Input: part model. Units: mm. Frame: model coordinates. A direction names the side the tool comes from. Give positions to 0.01 mm unless a question says otherwise; leave off trailing zeros. Loops run counter-clockwise (first coordinate to the right, second up) from the corner with the lowest first, then second, coordinate; pieces in that order, holes last. Notation, with made-up numbers: M 34.25,46.25 L 56.25,46.25 A22 ccw 56.25,75.25 Z; hole C 62.5,-11 d7. An arc over 180 degrees is marked long. Use CSV: the item, a comma, the result in double quotes. Start each with the question number.
Q1. Section A-A, the plane z = -11.5. Output: boundary loops of the cut face in (x, y), plus the area to 3 significant figures.
Q2. Pull-direction query (Z, two-part tool) for faces 3 (the flat face through (-7, -43, -20.32)), 4 (the conical face through (-6.28, -42.9, 26.58)), 5 (the flat face through (-25, -1, 15.24)); classes: released by +Z, released by -Z, zero draft, split by the parting line, or undercut.
Q3. Pin query (flat end, axial travel): pin 1 (10 mm diameter, centred on x = -38, y = -35.5, fed in from +Z); pin 2 (8 mm diameter, centred on x = -9, z = 3, fed in from +Y); pin 3 (1.5 mm diameter, centred on x = 49, z = 2, fed in from -Y); pin 4 (10 mm diameter, centred on x = -28, z = -15, fed in from -Y). Return the tip coordinate at first contact, or that it passes through.
Q4. Reachability of faces 1 (the flat face through (48, -5.08, 7)), 2 (the flat face through (-11, -5.08, 6)) from +Z, -Z, +X, -X, +Y, -Y: full face, straight path, thin tool, end or side. Return the list, or none.
Q5. Section B-B, the plane z = 29.5. Output: boundary loops of the cut face in (x, y).
Q6. Material intervals for line 1 along Y through (x, z) = (-14, -1); line 2 along Z through (x, y) = (1.5, -97); line 3 along Z through (x, y) = (-0.5, -57.5), sorted ascending.
from build123d import *

# Parameters (mm, degrees)
F1_ANGLE = 30
F2_T     = -5.08
F6_ANGLE = 1


with BuildPart() as f1:
    # F0 (on Front) → F1 (revolve)
    with BuildSketch(Plane.XZ):
        Polygon((-50.8, -20.32), (50.8, -20.32), (50.8, 20.32), (50.8, 33.02), (-50.8, 20.32), align=None)
    revolve(axis=Axis((-168.781414628, 0, 147.0986076593), (0, 0, -1)), revolution_arc=F1_ANGLE)

    # F2
    f2_openings = [f1.faces().sort_by_distance(p)[0] for p in [
        (43.317945, -56.831852, 6.35),
    ]]
    offset(amount=F2_T, openings=f2_openings, kind=Kind.INTERSECTION)

    # F3 (on face) → F4 (revolve, cut)
    with BuildSketch(Plane(origin=(0, 0, 0), x_dir=(-1, 0, 0), z_dir=(0, 1, 0))):
        Polygon((0, 0), (-45.72, 27.2654663298), (-45.72, -15.24), (0, -15.24), align=None)
    revolve(axis=Axis((-168.781414628, 0, 147.0986076593), (0, 0, -1)), mode=Mode.SUBTRACT)

    # F5 (on face) → F6 (revolve, cut)
    with BuildSketch(Plane.XZ):
        Polygon((-48.460111432, 15.24), (-48.460111432, 0), (0, 15.24), align=None)
    revolve(axis=Axis((-168.781414628, 0, 147.0986076593), (0, 0, -1)), revolution_arc=F6_ANGLE, mode=Mode.SUBTRACT)


solid = f1.part
A:
1,outline,"M -66.61,-58.99 L -22.61,-84.39 A168.78 ccw -20.14,-79.95 L -59.76,-57.08 A123.06 ccw -45.82,-5.08 L -0.08,-5.08 A168.78 ccw 0,0 L -50.8,0 A117.98 cw Z; M 16.98,-107.25 L 21.38,-109.79 A219.58 ccw 23.87,-105.36 L 19.47,-102.82 A214.5 cw Z; M 45.66,-5.08 L 50.74,-5.08 A219.58 ccw 50.8,0 L 45.72,0 A214.5 cw Z"
1,area,"837 mm^2"
2,face 3,"released by -Z"
2,face 4,"released by +Z"
2,face 5,"undercut"
3,pin 1,"z = 23.14"
3,pin 2,"y = 0"
3,pin 3,"y = -5.08"
3,pin 4,"y = -84.17"
4,face 1,"+X, -Y"
4,face 2,"+X"
5,outline,"M -3.01,-95.71 L 21.38,-109.79 A219.58 ccw 50.8,0 L 22.64,0 A191.42 cw Z"
6,line 1,"-5.08 to 0"
6,line 2,"-20.32 to -15.24, 16.21 to 30.07"
6,line 3,"-20.32 to -15.24, 22.68 to 27.8"
